Autodesk Inventor part; units mm, degrees
ref_plane "YZ Plane" through (0, 0, 0) normal (1, 0, 0) x (0, 1, 0)
ref_plane "XZ Plane" through (0, 0, 0) normal (0, 1, 0) x (-1, 0, 0)
ref_plane "XY Plane" through (0, 0, 0) normal (0, 0, 1) x (1, 0, 0)
sketch "Sketch1" plane through (0, 0, 0) normal (0, 1, 0) x (-1, 0, 0)
  line L0 (-30, 30) -> (30, 30)
  line L1 (30, 30) -> (30, -30)
  line L2 (30, -30) -> (-30, -30)
  line L3 (-30, -30) -> (-30, 30)
  line L4 (-31.35, 31.35) -> (31.35, 31.35)
  line L5 (31.35, 31.35) -> (31.35, -31.35)
  line L6 (31.35, -31.35) -> (-31.35, -31.35)
  line L7 (-31.35, -31.35) -> (-31.35, 31.35)
  line L8 (-35, 35) -> (35, 35)
  line L9 (35, 35) -> (35, -35)
  line L10 (35, -35) -> (-35, -35)
  line L11 (-35, -35) -> (-35, 35)
  point P0 (0, 0)
  point P1 (0, -30)
  point P2 (0, -31.35)
  point P3 (0, -35)
  point P4 (30, 0)
  point P5 (31.35, 0)
  point P6 (35, 0)
  dimension "d0" = 60
  dimension "d1" = 62.7
  dimension "d2" = 70
extrude "Extrusion1" add sketch "Sketch1" along normal blind 8 contours L4 L5 L6 L7
extrude "Extrusion2" add sketch "Sketch1" along normal blind 1 contours L8 L9 L10 L11
properties part number "VRSPAD-144 illumination base"
For this review, take the finished solid that the model builds, in its own axes (mm). A direction names the side the tool comes from. Give positions to 0.01 mm unless a question says otherwise; leave off trailing zeros. Write each loop counter-clockwise with the first axis right and the second up, starting at its lowest first coordinate (ties: lowest second). Pieces come first, ordered by that corner, then holes.
Item 1: Take a section at B-B (y = 3). Give the boundary of the cut face in (x, z).
Item 2: Machinability: for faces 1 (the face through (-31.35, 4, 0)), 2 (the face through (0, 4, -31.35)), 3 (the face through (0, 4, 30)), which of the approach directions +Z, -Z, +X, -X, +Y, -Y give a long, thin tool a straight path to every point of the face, cutting with its end or side? Answer none if there is none.
Item 3: Take a section at A-A (x = 14.5). Give the boundary of the cut face in (y, z), and give its area (3 significant figures).
Item 4: The part is to be moulded in two halves that separate along Z. For faces 4 (the face through (30.3, 8, 0.1)), 5 (the face through (0, 4, 31.35)), 6 (the face through (0, 4, -30)), say which applies: +Z half, -Z half, draft (parallel to the pull), parting line (faces both ways), or undercut.
Item 5: Take a section at C-C (z = 4.5). Give the boundary of the cut face in (x, y), and give its area (3 significant figures).
Item 6: Wall thickness on probe 1 along X at (y, z) = (4, -4); probe 2 along Z at (x, y) = (27.5, 0.75): over which ranges is each line inside the solid? List them lowest first.
Item 7: Insertion check: P1, Ø2, axis at x = -6, y = 6, coming from the +Z side; P2, Ø2, axis at x = -20, y = 3, coming from the -Z side; P3, Ø2, axis at y = 6, z = -8.5, coming from the -X side. Each pin has a flat end and moves straight along its axis. Give the tip position at first contact, or say it passes through.
Established:
1. outline: (-31.35, -31.35) - (31.35, -31.35) - (31.35, 31.35) - (-31.35, 31.35) - close; hole (-30, -30) - (30, -30) - (30, 30) - (-30, 30) - close
2. face 1: +Z, -Z, -X, +Y
2. face 2: -Z, +X, -X, +Y
2. face 3: +Y, -Y
3. outline: (0, -35) - (1, -35) - (1, -31.35) - (8, -31.35) - (8, -30) - (0, -30) - close; (0, 30) - (8, 30) - (8, 31.35) - (1, 31.35) - (1, 35) - (0, 35) - close
3. area: 28.9 mm2
4. face 4: draft
4. face 5: +Z half
4. face 6: undercut
5. outline: (-35, 0) - (-30, 0) - (-30, 8) - (-31.35, 8) - (-31.35, 1) - (-35, 1) - close; (30, 0) - (35, 0) - (35, 1) - (31.35, 1) - (31.35, 8) - (30, 8) - close
5. area: 28.9 mm2
6. probe 1: x = -31.35 to -30, 30 to 31.35
6. probe 2: z = -35 to -30, 30 to 35
7. P1: stops at z = 31.35
7. P2: stops at z = -31.35
7. P3: stops at x = -31.35
